Geometry: final body of the model. Coordinates: model frame, mm. A direction names the side the tool comes from. Coordinates: 2 decimals unless noted, no trailing zeros. Loops run counter-clockwise (first coordinate to the right, second up) from the corner with the lowest first, then second, coordinate; pieces in that order, holes last. Notation, with made-up numbers: (65.5, 72) - (98.5, 72) arc R17 ccw to (98.5, 103) - close; hole circle Ø10 at (-22, 64.25). An arc over 180 degrees is marked (long way). Put each result on its own line as item: value. Start each with the question number.
1) Reachability of faces 5 (the cylindrical face through (-9.021, 8.915, 0.178)), 6 (the cylindrical face through (13.843, 0.036, 0.178)), 7 (the cylindrical face through (14.86, -0.03, 0.18)) from +Z, -Z, +X, -X, +Y, -Y: full face, straight path, thin tool, end or side. Return the list, or none.
2) Contact query for a flat-ended pin moving along its axis: pin 1 Ø2 at (x, z) = (-1.5, -8) entering from +Y. Output: stop coordinate, or through.
3) Section B-B on x = 11. Output: boundary loops of the cut face in (y, z), and give its area (3 significant figures).
4) Section A-A on y = 0. Output: boundary loops of the cut face in (x, z), and give its area (3 significant figures).
5) Section C-C on y = 6.25. Output: boundary loops of the cut face in (x, z) (3 decimals).
6) Draft query along X for faces 1 (the flat face through (0, -6, 12.7)), 2 (the flat face through (0, -5.639, 0)), 3 (the cylindrical face through (-14.86, 0.03, 0.18)), 4 (the cylindrical face through (15.6, 8.9, 0.2)). Return one class per face: +X half, -X half, draft (parallel to the pull), parting line (faces both ways), or undercut.
7) Material intervals for line 1 along X through (y, z) = (7.75, -11.5) (3 decimals); line 2 along Y through (x, z) = (-11, 9); line 3 along X through (y, z) = (3.5, -2.5) (3 decimals), sorted ascending. Write a range as from..to.
```python
from build123d import *

# Parameters (mm, degrees)
BASE_EXTRUDE_DEPTH = 12.7


with BuildPart() as part:
    # Sketch1 → Base-Extrude (new, symmetric)
    with BuildSketch(Plane.XY):
        with BuildLine():
            Line((-15.875, 8.2042), (-15.875, 1.75976362))
            ThreePointArc((-15.875, 1.75976362), (-14.859, 0), (-15.875, -1.75976362))
            Line((-15.875, -1.75976362), (-15.875, -5.6388))
            ThreePointArc((-15.875, -5.6388), (-15.57742049, -6.35722049), (-14.859, -6.6548))
            Line((-14.859, -6.6548), (14.859, -6.6548))
            ThreePointArc((14.859, -6.6548), (15.57742049, -6.35722049), (15.875, -5.6388))
            Line((15.875, -5.6388), (15.875, -1.75976362))
            ThreePointArc((15.875, -1.75976362), (14.859, 0), (15.875, 1.75976362))
            Line((15.875, 1.75976362), (15.875, 8.2042))
            ThreePointArc((15.875, 8.2042), (15.57742049, 8.92262049), (14.859, 9.2202))
            Line((14.859, 9.2202), (9.74725, 9.2202))
            ThreePointArc((9.74725, 9.2202), (9.02882951, 8.92262049), (8.73125, 8.2042))
            Line((8.73125, 8.2042), (8.73125, 4.4577))
            Line((8.73125, 4.4577), (9.74725, 4.4577))
            Line((9.74725, 4.4577), (9.74725, 8.2042))
            Line((9.74725, 8.2042), (14.859, 8.2042))
            Line((14.859, 8.2042), (14.859, 2.271845065))
            ThreePointArc((14.859, 2.271845065), (13.843, 0), (14.859, -2.271845065))
            Line((14.859, -2.271845065), (14.859, -5.6388))
            Line((14.859, -5.6388), (-14.859, -5.6388))
            Line((-14.859, -5.6388), (-14.859, -2.271845065))
            ThreePointArc((-14.859, -2.271845065), (-13.843, 0), (-14.859, 2.271845065))
            Line((-14.859, 2.271845065), (-14.859, 8.2042))
            Line((-14.859, 8.2042), (-9.74725, 8.2042))
            Line((-9.74725, 8.2042), (-9.74725, 4.4577))
            Line((-9.74725, 4.4577), (-8.73125, 4.4577))
            Line((-8.73125, 4.4577), (-8.73125, 8.2042))
            ThreePointArc((-8.73125, 8.2042), (-9.02882951, 8.92262049), (-9.74725, 9.2202))
            Line((-9.74725, 9.2202), (-14.859, 9.2202))
            ThreePointArc((-14.859, 9.2202), (-15.57742049, 8.92262049), (-15.875, 8.2042))
        make_face()
    extrude(amount=BASE_EXTRUDE_DEPTH, both=True)


solid = part.part
```
Answer block:
1. face 5: +Z, -Z, +Y
1. face 6: +Z, -Z
1. face 7: +Z, -Z, +X
2. pin 1: stops at y = -5.64
3. outline: (-6.65, -12.7) - (-5.64, -12.7) - (-5.64, 12.7) - (-6.65, 12.7) - close; (8.2, -12.7) - (9.22, -12.7) - (9.22, 12.7) - (8.2, 12.7) - close
3. area: 51.6 mm²
4. outline: (-14.86, -12.7) - (-13.84, -12.7) - (-13.84, 12.7) - (-14.86, 12.7) - close; (13.84, -12.7) - (14.86, -12.7) - (14.86, 12.7) - (13.84, 12.7) - close
4. area: 51.6 mm²
5. outline: (-15.875, -12.7) - (-14.859, -12.7) - (-14.859, 12.7) - (-15.875, 12.7) - close; (-9.747, -12.7) - (-8.731, -12.7) - (-8.731, 12.7) - (-9.747, 12.7) - close; (8.731, -12.7) - (9.747, -12.7) - (9.747, 12.7) - (8.731, 12.7) - close; (14.859, -12.7) - (15.875, -12.7) - (15.875, 12.7) - (14.859, 12.7) - close
6. face 1: draft
6. face 2: undercut
6. face 3: -X half
6. face 4: +X half
7. line 1: x = -15.875..-14.859, -9.747..-8.731, 8.731..9.747, 14.859..15.875
7. line 2: y = -6.65..-5.64, 8.2..9.22
7. line 3: x = -15.875..-14.859, 14.859..15.875
